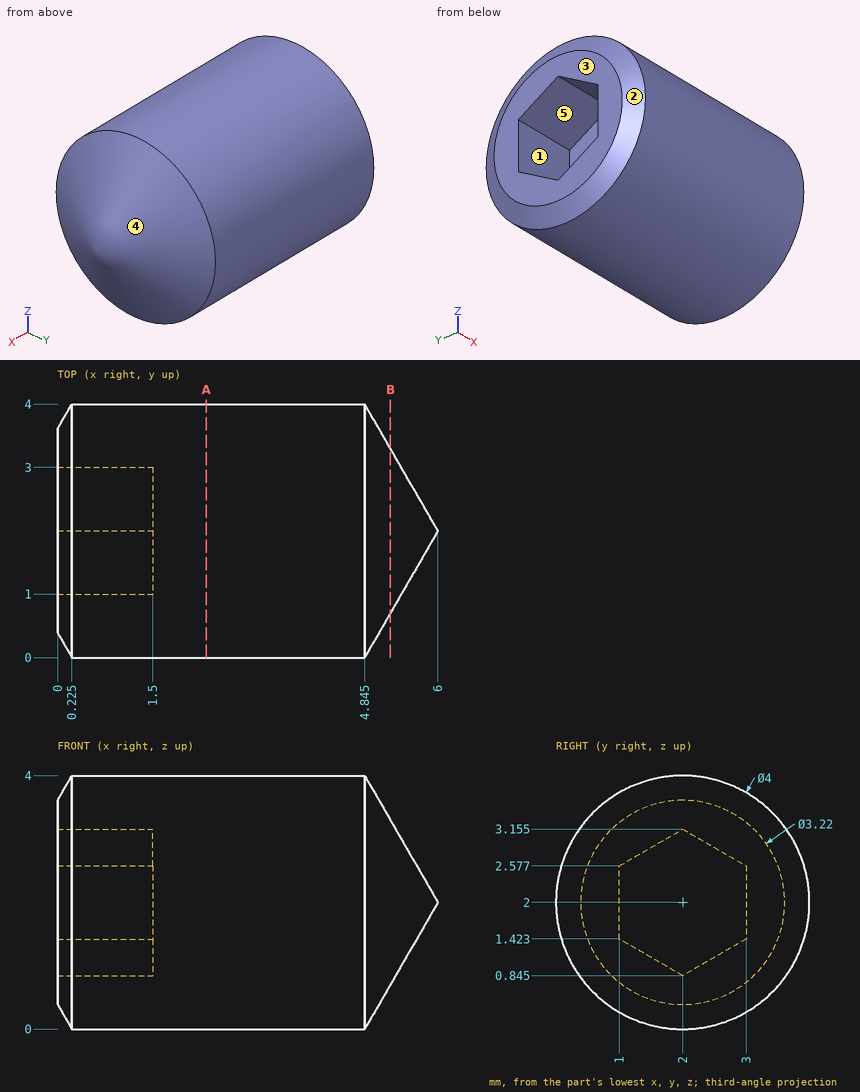
Source: three-view drawing plus pictorial views. Frame: mm from the lowest corner of the part. A direction names the side the tool comes from. Round coordinates to 2 decimals unless told otherwise and drop trailing zeros. Loops run counter-clockwise (first coordinate to the right, second up) from the corner with the lowest first, then second, coordinate; pieces in that order, holes last.
Item 1: Line query: L1, parallel to Z at x = 0.5, y = 1.25 (1 decimal); L2, parallel to Y at x = 1.4, z = 1.85 (1 decimal); L3, parallel to X at y = 1.8, z = 2.65. Output: solid intervals per line, ascending.
Checked values:
L1: z = 0.1 to 1.3, 2.7 to 3.9
L2: y = 0 to 1, 3 to 4
L3: x = 1.5 to 5.61
Item 2: Section B-B, the plane x = 5.25. Output: boundary loops of the cut face in (y, z).
Checked values:
outline: circle Ø2.6 at (2, 2)
Item 3: Mould query, pull axis Z, two halves, no side actions, for the marked faces 1, 2 and 3. Classes: released by +Z, released by -Z, zero draft, split by the parting line, or undercut.
Checked values:
face 1: undercut
face 2: split by the parting line
face 3: zero draft
Item 4: Section A-A, the plane x = 2.35. Output: boundary loops of the cut face in (y, z), plus the area to 3 significant figures.
Checked values:
outline: circle Ø4 at (2, 2)
area: 12.6 mm2
Item 5: Contact query for flat-ended pins moving along their axis: P1, Ø1, axis at x = 3, y = 3, coming from the -Z side; P2, Ø1.5, axis at x = 4.5, z = 1, coming from the -Y side; P3, Ø1.5, axis at x = 5.5, y = 1.5, coming from the -Z side (1 decimal). Output: stop coordinate, or through.
Checked values:
P1: stops at z = 0.06
P2: stops at y = 0.02
P3: stops at z = 0
Item 6: Reachability of the marked faces 4 and 5 from +Z, -Z, +X, -X, +Y, -Y: full face, straight path, thin tool, end or side. Return the list, or none.
Checked values:
face 4: +X
face 5: -X
